from build123d import *

# Parameters (mm, degrees)
SALIENTE_EXTRUIR1_DEPTH = 114
CROQUIS3_W              = 34.5
CROQUIS3_H              = 26.5
CORTAR_EXTRUIR1_DEPTH   = 111
CROQUIS4_W              = 40.5
CROQUIS4_H              = 7
CORTAR_EXTRUIR2_DEPTH   = 29.5
CROQUIS5_W              = 15
CROQUIS5_H              = 3
CORTAR_EXTRUIR3_DEPTH   = 122.096294328
CROQUIS6_R              = 1.75
CORTAR_EXTRUIR4_DEPTH   = 121.856578224
SALIENTE_EXTRUIR2_DEPTH = 3
CROQUIS8_R              = 1.75
CORTAR_EXTRUIR5_DEPTH   = 118.705083301
REDONDEO1_R             = 2


with BuildPart() as part:
    # Croquis1 → Saliente-Extruir1 (new body)
    with BuildSketch(Plane(origin=(0, 0, 0), x_dir=(1, 0, 0), z_dir=(0, 1, 0))):
        Polygon((0, 0), (-28.25, 0), (-28.25, 4), (-20.25, 4), (-20.25, 32.5), (20.25, 32.5), (20.25, 4), (28.25, 4), (28.25, 0), align=None)
    extrude(amount=SALIENTE_EXTRUIR1_DEPTH)

    # Croquis3 → Cortar-Extruir1 (cut)
    with BuildSketch(Plane(origin=(0, 114, 0), x_dir=(1, 0, 0), z_dir=(0, 1, 0))):
        with Locations((0, 16.25)):
            Rectangle(CROQUIS3_W, CROQUIS3_H)
    extrude(amount=-CORTAR_EXTRUIR1_DEPTH, mode=Mode.SUBTRACT)

    # Croquis4 → Cortar-Extruir2 (cut)
    with BuildSketch(Plane(origin=(0, 0, -32.5), x_dir=(-1, 0, 0), z_dir=(0, 0, -1))):
        with Locations((0, 110.5)):
            Rectangle(CROQUIS4_W, CROQUIS4_H)
    extrude(amount=-CORTAR_EXTRUIR2_DEPTH, mode=Mode.SUBTRACT)

    # Croquis5 → Cortar-Extruir3 (cut, through all)
    with BuildSketch(Plane(origin=(0, 0, -3), x_dir=(-1, 0, 0), z_dir=(0, 0, -1))):
        with Locations((0, 108.5)):
            Rectangle(CROQUIS5_W, CROQUIS5_H)
    extrude(amount=-CORTAR_EXTRUIR3_DEPTH, mode=Mode.SUBTRACT)

    # Croquis6 → Cortar-Extruir4 (cut, through all)
    with BuildSketch(Plane(origin=(0, 0, -4), x_dir=(-1, 0, 0), z_dir=(0, 0, -1))):
        with Locations((-24.25, 109.552589801)):
            Circle(CROQUIS6_R)
        with Locations((-24.25, 99.552589801)):
            Circle(CROQUIS6_R)
        with Locations((-24.25, 89.552589801)):
            Circle(CROQUIS6_R)
        with Locations((-24.25, 79.552589801)):
            Circle(CROQUIS6_R)
        with Locations((-24.25, 69.552589801)):
            Circle(CROQUIS6_R)
        with Locations((-24.25, 59.552589801)):
            Circle(CROQUIS6_R)
        with Locations((-24.25, 49.552589801)):
            Circle(CROQUIS6_R)
        with Locations((-24.25, 39.552589801)):
            Circle(CROQUIS6_R)
        with Locations((-24.25, 29.552589801)):
            Circle(CROQUIS6_R)
        with Locations((-24.25, 19.552589801)):
            Circle(CROQUIS6_R)
        with Locations((-24.25, 9.552589801)):
            Circle(CROQUIS6_R)
        with Locations(Location((24.25, 9.552589801, 0), (0, 0, 180))):
            Circle(CROQUIS6_R)
        with Locations(Location((24.25, 19.552589801, 0), (0, 0, 180))):
            Circle(CROQUIS6_R)
        with Locations(Location((24.25, 29.552589801, 0), (0, 0, 180))):
            Circle(CROQUIS6_R)
        with Locations(Location((24.25, 39.552589801, 0), (0, 0, 180))):
            Circle(CROQUIS6_R)
        with Locations(Location((24.25, 49.552589801, 0), (0, 0, 180))):
            Circle(CROQUIS6_R)
        with Locations(Location((24.25, 59.552589801, 0), (0, 0, 180))):
            Circle(CROQUIS6_R)
        with Locations(Location((24.25, 69.552589801, 0), (0, 0, 180))):
            Circle(CROQUIS6_R)
        with Locations(Location((24.25, 79.552589801, 0), (0, 0, 180))):
            Circle(CROQUIS6_R)
        with Locations(Location((24.25, 89.552589801, 0), (0, 0, 180))):
            Circle(CROQUIS6_R)
        with Locations(Location((24.25, 99.552589801, 0), (0, 0, 180))):
            Circle(CROQUIS6_R)
        with Locations(Location((24.25, 109.552589801, 0), (0, 0, 180))):
            Circle(CROQUIS6_R)
    extrude(amount=-CORTAR_EXTRUIR4_DEPTH, mode=Mode.SUBTRACT)

    # Croquis7 → Saliente-Extruir2 (add)
    with BuildSketch(Plane(origin=(0, 107, 0), x_dir=(1, 0, 0), z_dir=(0, 1, 0))):
        with BuildLine():
            Line((-4.257816839, 32.5), (-2.550631192, 38.239212117))
            ThreePointArc((-2.550631192, 38.239212117), (-0.065549886, 40.092694284), (2.41953142, 38.239212117))
            Line((2.41953142, 38.239212117), (4.126717066, 32.5))
            Line((4.126717066, 32.5), (-4.257816839, 32.5))
        make_face()
    extrude(amount=-SALIENTE_EXTRUIR2_DEPTH)

    # Croquis8 → Cortar-Extruir5 (cut, through all)
    with BuildSketch(Plane(origin=(0, 107, 0), x_dir=(1, 0, 0), z_dir=(0, 1, 0))):
        with Locations(Location((-0.065549886, 37.5, 0), (0, 0, 270))):
            Circle(CROQUIS8_R)
    extrude(amount=-CORTAR_EXTRUIR5_DEPTH, mode=Mode.SUBTRACT)

    # Redondeo1
    redondeo1_edges = [part.edges().sort_by_distance(p)[0] for p in [
        (0, 0, -32.5),
        (20.25, 0, -18.25),
        (-0.065549886, 104, -32.5),
        (4.126717066, 105.5, -32.5),
        (-4.257816839, 105.5, -32.5),
        (-17.25, 3, -16.25),
        (-20.25, 53.5, -32.5),
        (20.25, 53.5, -32.5),
    ]]
    fillet(redondeo1_edges, radius=REDONDEO1_R)


solid = part.part
Read the model definition and answer for the solid it produces. Units are mm, in the model's axes. A direction names the side the tool comes from. Coordinates: 2 decimals unless noted, no trailing zeros. Write each loop counter-clockwise with the first axis right and the second up, starting at its lowest first coordinate (ties: lowest second). Pieces come first, ordered by that corner, then holes. Notation, with made-up numbers: M -15.5,78.5 L 10.5,78.5 A29 ccw 10.5,106.5 Z; hole C 64,9 d6. An arc over 180 degrees is marked long. Use a Markdown table: item, result.
Q1. The part is cut by section D-D, the plane x = -24.25. Give the number of separate pieces and of enclosed holes in the cut face, then the cut area to 3 significant figures.
Answer block:
| item | result |
|---|---|
| separate pieces | 12 |
| enclosed holes | 0 |
| area | 302 mm2 |
Q2. Determine the mould class of faces 5 (the face through (24, 56, -4)), 6 (the face through (24.629, 17.844, -2.028)), 7 (the face through (-26, 59.5, -2)), 8 (the face through (-20.25, 53, -17)) for opening direction X: released by +X, released by -X, zero draft, split by the parting line, or undercut.
Answer block:
| item | result |
|---|---|
| face 5 | zero draft |
| face 6 | undercut |
| face 7 | undercut |
| face 8 | released by -X |
Q3. Straight lines are drawn through the part: L1, parallel to X at y = 67.5, z = -15.5; L2, parallel to Z at x = -3.5, y = 60.5; L3, parallel to Z at x = 17.5, y = 40. For each, find the intervals that lie inside material, in ascending order. Write a range as [from, to].
Answer block:
| item | result |
|---|---|
| L1 | x = [-20.25, -17.25], [17.25, 20.25] |
| L2 | z = [-32.5, -29.5], [-3, 0] |
| L3 | z = [-32.5, 0] |
Q4. The part is cut by section B-B, the plane y = 95. Write down the section's boundary in (x, z).
Answer block:
| item | result |
|---|---|
| outline | M -28.25,-4 L -20.25,-4 L -20.25,-30.5 A2 ccw -18.25,-32.5 L 18.25,-32.5 A2 ccw 20.25,-30.5 L 20.25,-4 L 28.25,-4 L 28.25,0 L -28.25,0 Z; hole M -17.25,-29.5 L 17.25,-29.5 L 17.25,-3 L -17.25,-3 Z |
Q5. Each of these flat-tipped pins is pushed along its axis until it touches: pin 1 Ø12 at (y, z) = (36.5, -26) entering from +X; pin 2 Ø5.5 at (x, y) = (24.25, 79.55) entering from -Z; pin 3 Ø12 at (x, y) = (-2, 70) entering from -Z. Where does it stop, or does it pass through?
Answer block:
| item | result |
|---|---|
| pin 1 | stops at x = 20.25 |
| pin 2 | stops at z = -4 |
| pin 3 | stops at z = -32.5 |
Q6. Which of the six approach directions +Z, -Z, +X, -X, +Y, -Y give full straight-line access (tool end or side, diameter ignored) to faces 1 (the face through (-24, 56, -4)), 2 (the face through (0, 56, -29.5)), 3 (the face through (3.052, 105.48, -36.115)), 4 (the face through (-7.5, 108, -2))?
Answer block:
| item | result |
|---|---|
| face 1 | -Z, -X, +Y, -Y |
| face 2 | +Y |
| face 3 | -Z, +X, +Y, -Y |
| face 4 | +Z, -Z |
Q7. The part is cut by section C-C, the plane z = -19.5. Write down the section's boundary in (x, y).
Answer block:
| item | result |
|---|---|
| outline | M -20.25,0 L 18.25,0 A2 ccw 20.25,2 L 20.25,107 L 17.25,107 L 17.25,3 L -15.25,3 A2 cw -17.25,5 L -17.25,107 L -20.25,107 Z |
Q8. The part is cut by section A-A, the plane x = 16. Write down the section's boundary in (y, z).
Answer block:
| item | result |
|---|---|
| outline | M 0,-30.5 A2 ccw 2,-32.5 L 107,-32.5 L 107,-29.5 L 3,-29.5 L 3,-3 L 114,-3 L 114,0 L 0,0 Z |
